from build123d import *

# Parameters (mm, degrees)
SFAZOWANIE1_SIZE           = 1
SZKIC5_W                   = 16
SZKIC5_H                   = 2
WYTNIJ_WYCI_GNI_CIE7_DEPTH = 39.691084286


with BuildPart() as part:
    # Szkic1 → Obrót1 (revolve)
    with BuildSketch(Plane.XY):
        with BuildLine():
            Line((0, 0), (5, 0))
            Line((5, 0), (5, 35.5))
            Line((5, 35.5), (8, 35.5))
            Line((8, 35.5), (8, 37))
            ThreePointArc((8, 37), (4.225307725, 39.017578445), (0, 39.7))
            Line((0, 39.7), (0, 0))
        make_face()
    revolve(axis=Axis((0, 0, 0), (0, 1, 0)))

    # Sfazowanie1
    sfazowanie1_edges = [part.edges().sort_by_distance(p)[0] for p in [
        (-5, 0, 0),
    ]]
    chamfer(sfazowanie1_edges, length=SFAZOWANIE1_SIZE)

    # Szkic5 → Wytnij-wyciągnięcie7 (cut, through all)
    with BuildSketch(Plane(origin=(0, 37, 0), x_dir=(1, 0, 0), z_dir=(0, 1, 0))):
        Rectangle(SZKIC5_W, SZKIC5_H)
    extrude(amount=WYTNIJ_WYCI_GNI_CIE7_DEPTH, mode=Mode.SUBTRACT)


solid = part.part
Can you work these out from the model? Positions are in its coordinate system, mm. A direction names the side the tool comes from. Coordinates: 2 decimals unless noted, no trailing zeros. Write each loop counter-clockwise with the first axis right and the second up, starting at its lowest first coordinate (ties: lowest second). Pieces come first, ordered by that corner, then holes. Notation, with made-up numbers: (62, 36.25) -> (107, 36.25) arc R9 ccw to (107, 47.25) -> close; hole circle Ø1 at (-31.75, 79). An arc over 180 degrees is marked (long way). Write each question's results on one line, items separated by ' | '. Start each with the question number.
Item 1: If we section it at A-A, the plane z = 0: Write out the boundary of the cut face in (x, y).
Item 2: Please list where these lines run through material, in increasing order: probe 1 along Z at (x, y) = (2.25, 35); probe 2 along Y at (x, z) = (0.75, -3.75); probe 3 along Y at (x, z) = (3.5, 0).
Item 3: Thinking about a two-plate mould opening in Z: for faces 3 (the cylindrical face through (-1.73, 36.26, 7.81)), 4 (the flat face through (0, 0, 0)), 5 (the flat face through (0, 37, 0)), which applies, released by +Z, released by -Z, zero draft, split by the parting line, or undercut?
Item 4: I'm going to push flat-ended pins straight in: P1, Ø4, axis at y = 18, z = -1.5, coming from the +X side; P2, Ø0.8, axis at x = -3.5, y = 38, coming from the -Z side; P3, Ø6, axis at y = 28.5, z = -5, coming from the -X side. Where does each tip first touch, or does it pass through?
Item 5: On a 3-axis mill with a long thin cutter (end or side, diameter ignored), from which of +Z, -Z, +X, -X, +Y, -Y can I reach the whole of each face in a straight line? I mean faces 1 (the flat face through (0.1, 35.5, 5.2)), 2 (the flat face through (0, 38, 1)). Say none if no direction works.
Item 6: If we section it at B-B, the plane y = 36.5: Write out the boundary of the cut face in (x, z).
Item 7: If we section it at C-C, the plane y = 32: Write out the boundary of the cut face in (x, z), and give its area (3 significant figures).
Answer block:
1) outline: (-8, 35.5) -> (-5, 35.5) -> (-5, 1) -> (-4, 0) -> (4, 0) -> (5, 1) -> (5, 35.5) -> (8, 35.5) -> (8, 37) -> (-8, 37) -> close
2) probe 1: -4.47 to 4.47 | probe 2: 0 to 39.15 | probe 3: 0 to 37
3) face 3: split by the parting line | face 4: zero draft | face 5: undercut
4) P1: x = 5 | P2: z = -6.27 | P3: x = -4.58
5) face 1: -Y | face 2: +X, -X, +Y
6) outline: circle Ø16 at (0, 0)
7) outline: circle Ø10 at (0, 0) | area: 78.5 mm²
